Read the model definition and answer for the solid it produces. Units are mm, in the model's axes. Face numbers are marked on the shaded views. A direction names the side the tool comes from. Give positions to 0.01 mm unless a question says otherwise; leave off trailing zeros. Order: outer loops, then holes, each group sorted by start corner. A loop starts at its lowest first (then second) coordinate and runs counter-clockwise, first axis right, second up. Notation, with made-up numbers: (49.25, 67) - (85.25, 67) arc R14 ccw to (85.25, 82) - close; hole circle Ø9 at (42, 45). An arc over 180 degrees is marked (long way). Write each question's results on one line, items separated by ' | '.
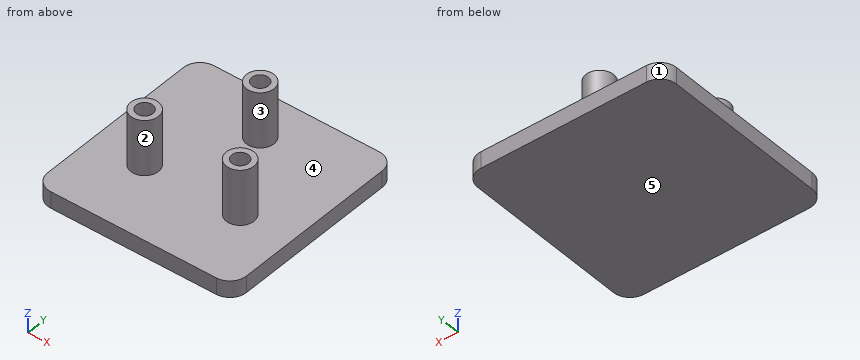
from build123d import *

# Parameters (mm, degrees)
SKETCH1_R           = 2.5
SKETCH1_R_2         = 1.5
BOSS_EXTRUDE1_DEPTH = 3
BOSS_EXTRUDE2_START = 3
SKETCH1_3_R         = 2.5
SKETCH1_3_R_2       = 1.5
BOSS_EXTRUDE2_DEPTH = 10


with BuildPart() as part:
    # Sketch1 → Boss-Extrude1 (new body)
    # profile 1 of 7: a face of its own
    with BuildSketch(Plane.XY):
        with BuildLine():
            ThreePointArc((-18, 15), (-17.121320344, 17.121320344), (-15, 18))
            Line((-15, 18), (15, 18))
            ThreePointArc((15, 18), (17.121320344, 17.121320344), (18, 15))
            Line((18, 15), (18, -15))
            ThreePointArc((18, -15), (17.121320344, -17.121320344), (15, -18))
            Line((15, -18), (-15, -18))
            ThreePointArc((-15, -18), (-17.121320344, -17.121320344), (-18, -15))
            Line((-18, -15), (-18, 15))
        make_face()
        with Locations((-8.660254038, -5)):
            Circle(SKETCH1_R, mode=Mode.SUBTRACT)
        with Locations((8.660254038, -5)):
            Circle(SKETCH1_R, mode=Mode.SUBTRACT)
        with Locations((0, 10)):
            Circle(SKETCH1_R, mode=Mode.SUBTRACT)
    # profile 2 of 7: a face of its own
    with BuildSketch(Plane.XY):
        with Locations((-8.660254038, -5)):
            Circle(SKETCH1_R)
        with Locations((-8.660254038, -5)):
            Circle(SKETCH1_R_2, mode=Mode.SUBTRACT)
    # profile 3 of 7: a face of its own
    with BuildSketch(Plane.XY):
        with Locations((-8.660254038, -5)):
            Circle(SKETCH1_R_2)
    # profile 4 of 7: a face of its own
    with BuildSketch(Plane.XY):
        with Locations((0, 10)):
            Circle(SKETCH1_R)
        with Locations((0, 10)):
            Circle(SKETCH1_R_2, mode=Mode.SUBTRACT)
    # profile 5 of 7: a face of its own
    with BuildSketch(Plane.XY):
        with Locations((0, 10)):
            Circle(SKETCH1_R_2)
    # profile 6 of 7: a face of its own
    with BuildSketch(Plane.XY):
        with Locations((8.660254038, -5)):
            Circle(SKETCH1_R)
        with Locations((8.660254038, -5)):
            Circle(SKETCH1_R_2, mode=Mode.SUBTRACT)
    # profile 7 of 7: a face of its own
    with BuildSketch(Plane.XY):
        with Locations((8.660254038, -5)):
            Circle(SKETCH1_R_2)
    extrude(amount=BOSS_EXTRUDE1_DEPTH)

    # Sketch1<3> → Boss-Extrude2 (add)
    # profile 1 of 3: a face of its own
    with BuildSketch(Plane.XY.offset(BOSS_EXTRUDE2_START)):
        with Locations((-8.660254038, -5)):
            Circle(SKETCH1_3_R)
        with Locations((-8.660254038, -5)):
            Circle(SKETCH1_3_R_2, mode=Mode.SUBTRACT)
    # profile 2 of 3: a face of its own
    with BuildSketch(Plane.XY.offset(BOSS_EXTRUDE2_START)):
        with Locations((0, 10)):
            Circle(SKETCH1_3_R)
        with Locations((0, 10)):
            Circle(SKETCH1_3_R_2, mode=Mode.SUBTRACT)
    # profile 3 of 3: a face of its own
    with BuildSketch(Plane.XY.offset(BOSS_EXTRUDE2_START)):
        with Locations((8.660254038, -5)):
            Circle(SKETCH1_3_R)
        with Locations((8.660254038, -5)):
            Circle(SKETCH1_3_R_2, mode=Mode.SUBTRACT)
    extrude(amount=BOSS_EXTRUDE2_DEPTH)


solid = part.part
(1) Consider probe 1 along Y at (x, z) = (0, 7.5); probe 2 along Z at (x, y) = (-7, -13); probe 3 along Y at (x, z) = (7.5, 11). Determine where each line is inside the solid, lowest interval first. Write a range as [from, to].
Conclusion:
probe 1: [7.5, 8.5], [11.5, 12.5] | probe 2: [0, 3] | probe 3: [-7.21, -5.95], [-4.05, -2.79]
(2) For the marked faces 4 and 5, determine the directions among +Z, -Z, +X, -X, +Y, -Y from which every point of the face is accessible in a straight line to the end or side of a thin tool.
Conclusion:
face 4: +Z | face 5: -Z, +X, -X, +Y, -Y
(3) Section A-A (z = 9.75) is taken. Give the vertices of the cut face in (x, y).
Conclusion:
outline: circle Ø5 at (-8.66, -5); circle Ø5 at (0, 10); circle Ø5 at (8.66, -5); hole circle Ø3 at (-8.66, -5); hole circle Ø3 at (0, 10); hole circle Ø3 at (8.66, -5)
(4) Section C-C (x = 0) is taken. Give the vertices of the cut face in (y, z), plus the area to 3 significant figures.
Conclusion:
outline: (-18, 0) - (18, 0) - (18, 3) - (12.5, 3) - (12.5, 13) - (11.5, 13) - (11.5, 3) - (8.5, 3) - (8.5, 13) - (7.5, 13) - (7.5, 3) - (-18, 3) - close | area: 128 mm^2
(5) Section B-B (y = 10) is taken. Give the vertices of the cut face in (x, z), plus the area to 3 significant figures.
Conclusion:
outline: (-18, 0) - (18, 0) - (18, 3) - (2.5, 3) - (2.5, 13) - (1.5, 13) - (1.5, 3) - (-1.5, 3) - (-1.5, 13) - (-2.5, 13) - (-2.5, 3) - (-18, 3) - close | area: 128 mm^2
(6) The mould has two halves that part along X. Classify the marked faces 1, 2 and 3: pulls with the +X half, pulls with the -X half, needs draft (parallel to the pull), parting line crosses it, or undercut.
Conclusion:
face 1: pulls with the -X half | face 2: undercut | face 3: parting line crosses it
(7) Each of these flat-tipped pins is pushed along its axis until it touches: pin 1 (5 mm diameter, centred on x = 7, y = -13.5, fed in from +Z); pin 2 (3.5 mm diameter, centred on x = 9, y = -4.5, fed in from +Z); pin 3 (2 mm diameter, centred on x = -9.5, z = 8.5, fed in from -Y); pin 4 (4 mm diameter, centred on x = -2.5, z = 11, fed in from +Y). Where does it stop, or does it pass through?
Conclusion:
pin 1: z = 3 | pin 2: z = 13 | pin 3: y = -7.5 | pin 4: y = 12.45
(8) Section D-D (x = -13) is taken. Give the vertices of the cut face in (y, z).
Conclusion:
outline: (-18, 0) - (18, 0) - (18, 3) - (-18, 3) - close
